```python
from build123d import *

# Parameters (mm, degrees)
F2_R     = 11.95
F3_DEPTH = 72.45
F4_R     = 7.7
F5_DEPTH = 5.001


with BuildPart() as f1:
    # F0 (on Front) → F1 (revolve)
    with BuildSketch(Plane.XZ):
        Polygon((-34.341893, 12.8), (-34.341893, 0), (40.508107, 0), (40.508107, 10.6), (43.108107, 12.5), (43.108107, 14.1), (20.658107, 14.1), (18.408107, 13.4), (-21.741893, 13.4), (-24.141893, 15.3), (-27.041893, 15.3), (-27.041893, 12.8), align=None)
    revolve(axis=Axis((3.083107, 0, 0), (-1, 0, 0)))

    # F2 (on face) → F3 (cut)
    with BuildSketch(Plane(origin=(-34.341893, 0, 0), x_dir=(0, -1, 0), z_dir=(-1, 0, 0))):
        Circle(F2_R)
    extrude(amount=-F3_DEPTH, mode=Mode.SUBTRACT)

    # F4 (on face) → F5 (cut, through all)
    with BuildSketch(Plane(origin=(38.108107, 0, 0), x_dir=(0, -1, 0), z_dir=(-1, 0, 0))):
        Circle(F4_R)
    extrude(amount=-F5_DEPTH, mode=Mode.SUBTRACT)


solid = f1.part
```
Design review of the part built by this model. Coordinates are the model's own, in mm. A direction names the side the tool comes from. Give positions to 0.01 mm unless a question says otherwise; leave off trailing zeros. Order: outer loops, then holes, each group sorted by start corner. A loop starts at its lowest first (then second) coordinate and runs counter-clockwise, first axis right, second up. Notation, with made-up numbers: M 22.5,44 L 45.5,44 A25 cw 45.5,68 Z; hole C -16,54.5 d9. An arc over 180 degrees is marked long. One line per question, with ' | ' between items. Start each with the question number.
Q1. The part is to be moulded in two halves that separate along X. For faces 5 (the face through (38.108, 0, -8)), 6 (the face through (-21.892, -13.197, -2.931)), 7 (the face through (43.108, -12.5, 2.2)), say which applies: +X half, -X half, draft (parallel to the pull), parting line (faces both ways), or undercut.
Q2. For pin 1 Ø1 at (x, z) = (13.5, 12) entering from -Y; pin 2 Ø1 at (x, z) = (32.5, -1.5) entering from +Y; pin 3 Ø12 at (x, z) = (0, 4.5) entering from +Y, all flat-tipped, find the tip position at first contact; note any pin that passes through.
Q3. We need section A-A (z = 0). Write out the cut boundary in (x, y).
Q4. For L1, parallel to Z at x = 3, y = 10; L2, parallel to Z at x = -11.5, y = -7.5; L3, parallel to Y at x = 4.5, z = -4, list the stretches that pass through material, from the lowest coordinate up. Write a range as [from, to].
Q5. We need section C-C (x = 16). Write out the cut boundary in (y, z).
Q6. Machinability: for faces 1 (the face through (-30.743, -7.789, -10.158)), 2 (the face through (31.726, -12.509, 6.506)), 3 (the face through (-1.948, 0.589, -13.387)), 4 (the face through (39.291, 1.669, -7.517)), which of the approach directions +Z, -Z, +X, -X, +Y, -Y give a long, thin tool a straight path to every point of the face, cutting with its end or side? Answer none if there is none.
Q7. We need section D-D (x = -25). Write out the cut boundary in (y, z), plus the area to 3 significant figures.
Returned:
1) face 5: -X half | face 6: undercut | face 7: +X half
2) pin 1: y = -6.88 | pin 2: y = 14.06 | pin 3: y = 13.4
3) outline: M -34.34,-12.8 L -27.04,-12.8 L -27.04,-15.3 L -24.14,-15.3 L -21.74,-13.4 L 18.41,-13.4 L 20.66,-14.1 L 43.11,-14.1 L 43.11,-12.5 L 40.51,-10.6 L 40.51,-7.7 L 38.11,-7.7 L 38.11,-11.95 L -34.34,-11.95 Z; M -34.34,11.95 L 38.11,11.95 L 38.11,7.7 L 40.51,7.7 L 40.51,10.6 L 43.11,12.5 L 43.11,14.1 L 20.66,14.1 L 18.41,13.4 L -21.74,13.4 L -24.14,15.3 L -27.04,15.3 L -27.04,12.8 L -34.34,12.8 Z
4) L1: [-8.92, -6.54], [6.54, 8.92] | L2: [-11.1, -9.3], [9.3, 11.1] | L3: [-12.79, -11.26], [11.26, 12.79]
5) outline: C 0,0 d26.8; hole C 0,0 d23.9
6) face 1: -X | face 2: +X | face 3: none | face 4: +X, -X
7) outline: C 0,0 d30.6; hole C 0,0 d23.9 | area: 287 mm2
